from build123d import *

# Parameters (mm, degrees)
BOSS_EXTRUDE1_DEPTH = 1
SKETCH1_3_R         = 1.5
BOSS_EXTRUDE2_DEPTH = 2


with BuildPart() as part:
    # Sketch1 → Boss-Extrude1 (new body)
    with BuildSketch(Plane.XY):
        with BuildLine():
            Line((8.045815072, 27.495269935), (-0.183811683, 30.090061284))
            ThreePointArc((-0.183811683, 30.090061284), (-17.81741665, 47.650937168), (6.207550462, 41.160225249))
            Line((6.207550462, 41.160225249), (12.569519065, 35.330555089))
            ThreePointArc((12.569519065, 35.330555089), (13.331800916, 34.427699543), (13.84093453, 33.361395308))
            Line((13.84093453, 33.361395308), (13.081997543, 29.050910113))
            ThreePointArc((13.081997543, 29.050910113), (10.806658392, 27.487211768), (8.045815072, 27.495269935))
        make_face()
    extrude(amount=-BOSS_EXTRUDE1_DEPTH)

    # Sketch1_3 → Boss-Extrude2 (add)
    with BuildSketch(Plane.XY):
        with BuildLine():
            Line((14.790918873, 33.673692842), (18.278866438, 31.659925376))
            Line((18.278866438, 31.659925376), (15.778866438, 27.329798357))
            Line((15.778866438, 27.329798357), (13.868189747, 28.432928059))
            ThreePointArc((13.868189747, 28.432928059), (11.101791823, 26.531755721), (7.745109273, 26.541552984))
            Line((7.745109273, 26.541552984), (-0.071885696, 29.006242031))
            ThreePointArc((-0.071885696, 29.006242031), (-18.683442054, 48.150937168), (7.202128462, 41.605204128))
            Line((7.202128462, 41.605204128), (13.245109273, 36.067832426))
            ThreePointArc((13.245109273, 36.067832426), (14.171905143, 34.970124549), (14.790918873, 33.673692842))
        make_face()
        with BuildLine():
            ThreePointArc((8.045815072, 27.495269935), (10.806658392, 27.487211768), (13.081997543, 29.050910113))
            Line((13.081997543, 29.050910113), (13.84093453, 33.361395308))
            ThreePointArc((13.84093453, 33.361395308), (13.331800916, 34.427699543), (12.569519065, 35.330555089))
            Line((12.569519065, 35.330555089), (6.207550462, 41.160225249))
            ThreePointArc((6.207550462, 41.160225249), (-17.81741665, 47.650937168), (-0.183811683, 30.090061284))
            Line((-0.183811683, 30.090061284), (8.045815072, 27.495269935))
        make_face(mode=Mode.SUBTRACT)
        with BuildLine():
            Line((8.045815072, 27.495269935), (-0.183811683, 30.090061284))
            ThreePointArc((-0.183811683, 30.090061284), (-17.81741665, 47.650937168), (6.207550462, 41.160225249))
            Line((6.207550462, 41.160225249), (12.569519065, 35.330555089))
            ThreePointArc((12.569519065, 35.330555089), (13.331800916, 34.427699543), (13.84093453, 33.361395308))
            Line((13.84093453, 33.361395308), (13.081997543, 29.050910113))
            ThreePointArc((13.081997543, 29.050910113), (10.806658392, 27.487211768), (8.045815072, 27.495269935))
        make_face()
        with BuildLine():
            Line((24.429975611, 42.313958986), (0.94372521, 55.144959619))
            ThreePointArc((0.94372521, 55.144959619), (-20.908315232, 48.228438049), (-13.073721217, 26.688496574))
            Line((-13.073721217, 26.688496574), (9.627757266, 16.675764747))
            Line((9.627757266, 16.675764747), (15.778866438, 27.329798357))
            Line((15.778866438, 27.329798357), (13.868189747, 28.432928059))
            ThreePointArc((13.868189747, 28.432928059), (11.101791823, 26.531755721), (7.745109273, 26.541552984))
            Line((7.745109273, 26.541552984), (-0.071885696, 29.006242031))
            ThreePointArc((-0.071885696, 29.006242031), (-18.683442054, 48.150937168), (7.202128462, 41.605204128))
            Line((7.202128462, 41.605204128), (13.245109273, 36.067832426))
            ThreePointArc((13.245109273, 36.067832426), (14.171905143, 34.970124549), (14.790918873, 33.673692842))
            Line((14.790918873, 33.673692842), (18.278866438, 31.659925376))
            Line((18.278866438, 31.659925376), (24.429975611, 42.313958986))
        make_face()
        with Locations((4.709200809, 23.09818313)):
            Circle(SKETCH1_3_R, mode=Mode.SUBTRACT)
        with Locations((15.709200809, 42.150742014)):
            Circle(SKETCH1_3_R, mode=Mode.SUBTRACT)
    extrude(amount=BOSS_EXTRUDE2_DEPTH)


solid = part.part
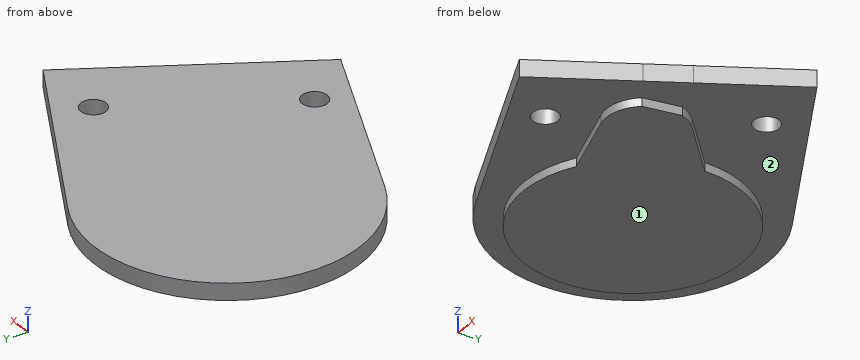
The listing builds one solid part. Answer for the finished solid, in the listing's coordinates (mm). Face numbers are marked on the shaded views. A direction names the side the tool comes from. Coordinates: 2 decimals unless noted, no trailing zeros. Order: outer loops, then holes, each group sorted by start corner. A loop starts at its lowest first (then second) coordinate and runs counter-clockwise, first axis right, second up. Notation, with made-up numbers: (54, -2) -> (96, -2) arc R29 ccw to (96, 37) -> close; hole circle Ø4 at (16.25, 34). An arc over 180 degrees is marked (long way). Answer in a Markdown table with one row per item. Add a question column.
Item 1: Find section A-A (y = 43). Write down the section's boundary in (x, z).
Item 2: Find section D-D (x = -7). Write down the section's boundary in (y, z), then the cut area to 3 significant figures.
Item 3: Which of the six approach directions +Z, -Z, +X, -X, +Y, -Y give full straight-line access (tool end or side, diameter ignored) to the marked faces 1 and 2?
Item 4: Find section C-C (z = 1.4). State how many separate pieces and enclosed holes the cut face has, then the cut area to 3 significant figures.
Item 5: Find the intervals of material crossed by L1, parallel to Z at x = 11, y = 47; L2, parallel to X at y = 23, z = 0.6; L3, parallel to Y at x = 0, z = 1.1, in increasing order. Write a range as from..to.
Item 6: This flat-tipped pin is pushed along its axis until it touches: P1, Ø5, axis at x = 15.71, y = 42.15, coming from the -Z side. Where does it stop, or does it pass through?
Item 7: Find section B-B (x = 4.5). Write down the section's boundary in (y, z), then the cut area to 3 significant figures.
Result set:
| question | item | result |
|---|---|---|
| 1 | outline | (-22.44, 0) -> (-19.42, 0) -> (-19.42, -1) -> (6.08, -1) -> (6.08, 0) -> (14.47, 0) -> (14.47, 2) -> (-22.44, 2) -> close; (16.95, 0) -> (23.17, 0) -> (23.17, 2) -> (16.95, 2) -> close |
| 2 | outline | (24.01, 0) -> (28.34, 0) -> (28.34, -1) -> (54.08, -1) -> (54.08, 0) -> (57.08, 0) -> (57.08, 2) -> (24.01, 2) -> close |
| 2 | area | 91.9 mm² |
| 3 | face 1 | -Z, +X, -X, +Y, -Y |
| 3 | face 2 | -Z |
| 4 | separate pieces | 1 |
| 4 | enclosed holes | 2 |
| 4 | area | 1,190 mm² |
| 5 | L1 | z = 0..2 |
| 5 | L2 | x = -4.71..3.21, 6.21..13.28 |
| 5 | L3 | y = 20.92..55.62 |
| 6 | P1 | stops at z = 0 |
| 7 | outline | (18.94, 0) -> (21.61, 0) -> (21.61, 2) -> (18.94, 2) -> close; (24.58, 0) -> (28.61, 0) -> (28.61, -1) -> (47.62, -1) -> (47.62, 0) -> (53.2, 0) -> (53.2, 2) -> (24.58, 2) -> close |
| 7 | area | 81.6 mm² |
